Verification items for the finished model (mm, model axes). Face numbers are marked on the shaded views. A direction names the side the tool comes from. Round coordinates to 2 decimals unless told otherwise and drop trailing zeros. Loops run counter-clockwise (first coordinate to the right, second up) from the corner with the lowest first, then second, coordinate; pieces in that order, holes last. Notation, with made-up numbers: (-27.75, 30) - (24.25, 30) arc R17 ccw to (24.25, 62) - close; hole circle Ø1 at (59, 89.25). An arc over 180 degrees is marked (long way). Use a Markdown table: item, result. Add a question column.
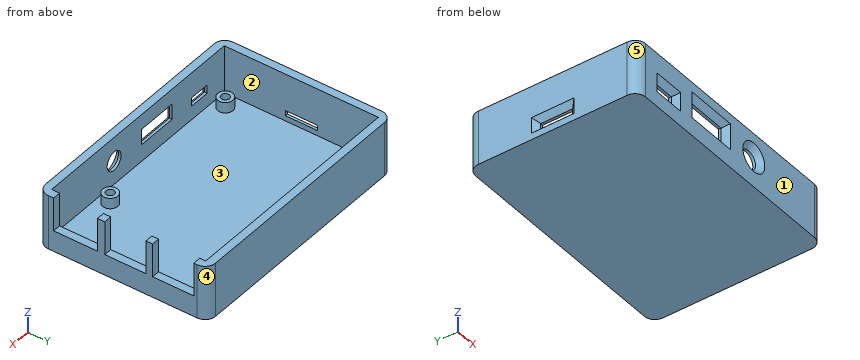
```python
from build123d import *

# Parameters (mm, degrees)
BASE_SKETCH_W               = 93
BASE_SKETCH_H               = 64
BASE_DEPTH                  = 2.5
WALLS_SKETCH_W              = 93
WALLS_SKETCH_H              = 64
WALLS_SKETCH_W_2            = 87
WALLS_SKETCH_H_2            = 58
WALLS_DEPTH                 = 18
FRONT_CONNECTORS_REACH      = 102.465
FRONT_CONNECTORS_SKETCH_W   = 12.6
FRONT_CONNECTORS_SKETCH_H   = 16.5
FRONT_CONNECTORS_SKETCH_H_2 = 15.5
SIDE_CONNECTORS_REACH       = 83.722
SIDE_CONNECTORS_SKETCH_R    = 3.5
SIDE_CONNECTORS_SKETCH_W    = 8
SIDE_CONNECTORS_SKETCH_H    = 3.2
SIDE_CONNECTORS_SKETCH_W_2  = 15.3
SIDE_CONNECTORS_SKETCH_H_2  = 5.9
SIDE_CONNECTORS_ANGLE_SIZE  = 2
SD_SLOT_REACH               = 102.465
SD_SLOT_SKETCH_W            = 2
SD_SLOT_SKETCH_H            = 12
SD_SLOT_ANGLE_SIZE          = 2
MOUNT_PILLAR_SKETCH_R       = 2.85
MOUNT_PILLARS_DEPTH         = 4
INSERT_NUT_HOLES_D          = 3.1
INSERT_NUT_HOLES_DEPTH      = 5
INSERT_NUT_HOLES_TIP        = 0.931333959
ZAOBLIT2_R                  = 4


with BuildPart() as part:
    # Base sketch → Base (new body)
    with BuildSketch(Plane.XY):
        Rectangle(BASE_SKETCH_W, BASE_SKETCH_H)
    extrude(amount=BASE_DEPTH)

    # Walls sketch → Walls (add)
    with BuildSketch(Plane.XY.offset(2.5)):
        Rectangle(WALLS_SKETCH_W, WALLS_SKETCH_H)
        Rectangle(WALLS_SKETCH_W_2, WALLS_SKETCH_H_2, mode=Mode.SUBTRACT)
    extrude(amount=WALLS_DEPTH)

    # Front connectors sketch → Front connectors (cut, up to next)
    with BuildSketch(Plane(origin=(46.5, 0, 0), x_dir=(0, 0, -1), z_dir=(1, 0, 0)), mode=Mode.PRIVATE) as front_connectors_sk1:
        with Locations((-14.2, -17.75)):
            Rectangle(FRONT_CONNECTORS_SKETCH_W, FRONT_CONNECTORS_SKETCH_H)
    front_connectors_tool1 = extrude(front_connectors_sk1.sketch, amount=-FRONT_CONNECTORS_REACH, mode=Mode.PRIVATE) & part.part
    # Front connectors sketch → Front connectors (cut, up to next)
    with BuildSketch(Plane(origin=(46.5, 0, 0), x_dir=(0, 0, -1), z_dir=(1, 0, 0)), mode=Mode.PRIVATE) as front_connectors_sk2:
        with Locations((-14.2, 1)):
            Rectangle(FRONT_CONNECTORS_SKETCH_W, FRONT_CONNECTORS_SKETCH_H_2)
    front_connectors_tool2 = extrude(front_connectors_sk2.sketch, amount=-FRONT_CONNECTORS_REACH, mode=Mode.PRIVATE) & part.part
    # Front connectors sketch → Front connectors (cut, up to next)
    with BuildSketch(Plane(origin=(46.5, 0, 0), x_dir=(0, 0, -1), z_dir=(1, 0, 0)), mode=Mode.PRIVATE) as front_connectors_sk3:
        with Locations((-14.2, 19)):
            Rectangle(FRONT_CONNECTORS_SKETCH_W, FRONT_CONNECTORS_SKETCH_H_2)
    front_connectors_tool3 = extrude(front_connectors_sk3.sketch, amount=-FRONT_CONNECTORS_REACH, mode=Mode.PRIVATE) & part.part
    add(front_connectors_tool1.solids().sort_by_distance((46.5, -17.75, 14.2))[0], mode=Mode.SUBTRACT)
    add(front_connectors_tool2.solids().sort_by_distance((46.5, 1, 14.2))[0], mode=Mode.SUBTRACT)
    add(front_connectors_tool3.solids().sort_by_distance((46.5, 19, 14.2))[0], mode=Mode.SUBTRACT)

    # Side connectors sketch → Side connectors (cut, up to next)
    with BuildSketch(Plane.XZ.offset(32), mode=Mode.PRIVATE) as side_connectors_sk1:
        with Locations(Location((12, 11.4, 0), (0, 0, 270))):
            Circle(SIDE_CONNECTORS_SKETCH_R)
    side_connectors_tool1 = extrude(side_connectors_sk1.sketch, amount=-SIDE_CONNECTORS_REACH, mode=Mode.PRIVATE) & part.part
    # Side connectors sketch → Side connectors (cut, up to next)
    with BuildSketch(Plane.XZ.offset(32), mode=Mode.PRIVATE) as side_connectors_sk2:
        with Locations((-30.9, 9.3)):
            Rectangle(SIDE_CONNECTORS_SKETCH_W, SIDE_CONNECTORS_SKETCH_H)
    side_connectors_tool2 = extrude(side_connectors_sk2.sketch, amount=-SIDE_CONNECTORS_REACH, mode=Mode.PRIVATE) & part.part
    # Side connectors sketch → Side connectors (cut, up to next)
    with BuildSketch(Plane.XZ.offset(32), mode=Mode.PRIVATE) as side_connectors_sk3:
        with Locations((-9.5, 11.85)):
            Rectangle(SIDE_CONNECTORS_SKETCH_W_2, SIDE_CONNECTORS_SKETCH_H_2)
    side_connectors_tool3 = extrude(side_connectors_sk3.sketch, amount=-SIDE_CONNECTORS_REACH, mode=Mode.PRIVATE) & part.part
    add(side_connectors_tool1.solids().sort_by_distance((12, -32, 11.4))[0], mode=Mode.SUBTRACT)
    add(side_connectors_tool2.solids().sort_by_distance((-30.9, -32, 9.3))[0], mode=Mode.SUBTRACT)
    add(side_connectors_tool3.solids().sort_by_distance((-9.5, -32, 11.85))[0], mode=Mode.SUBTRACT)

    # Side connectors angle
    side_connectors_angle_edges = [part.edges().sort_by_distance(p)[0] for p in [
        (-9.5, -32, 8.9),
        (-1.85, -32, 11.85),
        (-9.5, -32, 14.8),
        (-17.15, -32, 11.85),
        (12, -32, 14.9),
        (-34.9, -32, 9.3),
        (-30.9, -32, 7.7),
        (-26.9, -32, 9.3),
        (-30.9, -32, 10.9),
    ]]
    chamfer(side_connectors_angle_edges, length=SIDE_CONNECTORS_ANGLE_SIZE)

    # SD slot sketch → SD slot (cut, up to next)
    with BuildSketch(Plane.ZY.offset(46.5), mode=Mode.PRIVATE) as sd_slot_sk1:
        with Locations((5.5, 0)):
            Rectangle(SD_SLOT_SKETCH_W, SD_SLOT_SKETCH_H)
    sd_slot_tool1 = extrude(sd_slot_sk1.sketch, amount=-SD_SLOT_REACH, mode=Mode.PRIVATE) & part.part
    add(sd_slot_tool1.solids().sort_by_distance((-46.5, 0, 5.5))[0], mode=Mode.SUBTRACT)

    # SD slot angle
    sd_slot_angle_edges = [part.edges().sort_by_distance(p)[0] for p in [
        (-46.5, 0, 6.5),
        (-46.5, -6, 5.5),
        (-46.5, 6, 5.5),
        (-46.5, 0, 4.5),
    ]]
    chamfer(sd_slot_angle_edges, length=SD_SLOT_ANGLE_SIZE)

    # Mount pillar sketch → Mount pillars (add)
    with BuildSketch(Plane.XY.offset(2.5)):
        with Locations((-38, -24.5)):
            Circle(MOUNT_PILLAR_SKETCH_R)
        with Locations((20, -24.5)):
            Circle(MOUNT_PILLAR_SKETCH_R)
        with Locations((20, 24.5)):
            Circle(MOUNT_PILLAR_SKETCH_R)
        with Locations((-38, 24.5)):
            Circle(MOUNT_PILLAR_SKETCH_R)
    extrude(amount=MOUNT_PILLARS_DEPTH)

    # Insert nut holes
    with Locations(Plane.XY.offset(6.5)):
        with Locations((-38, 24.5), (20, 24.5), (20, -24.5), (-38, -24.5)):
            Hole(INSERT_NUT_HOLES_D / 2, depth=INSERT_NUT_HOLES_DEPTH)
            with Locations((0, 0, -(INSERT_NUT_HOLES_DEPTH + INSERT_NUT_HOLES_TIP / 2))):  # 118° drill point
                Cone(0, INSERT_NUT_HOLES_D / 2, INSERT_NUT_HOLES_TIP, mode=Mode.SUBTRACT)

    # Zaoblit2
    zaoblit2_edges = [part.edges().sort_by_distance(p)[0] for p in [
        (46.5, 32, 10.25),
        (46.5, -32, 10.25),
        (-46.5, -32, 10.25),
        (-46.5, 32, 10.25),
    ]]
    fillet(zaoblit2_edges, radius=ZAOBLIT2_R)


solid = part.part
```
Q1. Section check D-D on y = -12.5. Record the cut outline in (x, z).
Q2. Section check A-A on y = 1. Record the cut outline in (x, z), plus the area to 3 significant figures.
Q3. Section check C-C on z = 19.25. Record the cut outline in (x, y).
Q4. Section check B-B on x = 12. Record the cut outline in (y, z), plus the area to 3 significant figures.
Q5. Go/stop test with flat-tipped pins: pin 1 Ø0.8 at (y, z) = (-29.5, 12) entering from -X; pin 2 Ø6 at (y, z) = (4, 14.5) entering from +X; pin 3 Ø2.5 at (x, z) = (45, 12.5) entering from +Y. Record where each tip stops, or that it passes through.
Q6. Set-up check for the marked faces 1 and 2: record each of +Z, -Z, +X, -X, +Y, -Y from which the full face is reachable in a straight line by a thin tool's end or side.
Q7. Thickness scan on line 1 along Y through (x, z) = (-38, 3.7); line 2 along Y through (x, z) = (30, 17.75); line 3 along X through (y, z) = (11.5, 5.5). Record the ranges inside material, lowest first.
Q8. Release check for a two-part mould opening along X. For the marked faces 3, 4 and 5 record: +X half, -X half, draft (parallel to the pull), parting line (faces both ways), or undercut.
Determined:
| question | item | result |
|---|---|---|
| 1 | outline | (-46.5, 0) - (46.5, 0) - (46.5, 7.9) - (43.5, 7.9) - (43.5, 2.5) - (-43.5, 2.5) - (-43.5, 20.5) - (-46.5, 20.5) - close |
| 2 | outline | (-46.5, 0) - (46.5, 0) - (46.5, 7.9) - (43.5, 7.9) - (43.5, 2.5) - (-43.5, 2.5) - (-43.5, 4.5) - (-44.5, 4.5) - (-46.5, 2.5) - close; (-46.5, 8.5) - (-44.5, 6.5) - (-43.5, 6.5) - (-43.5, 20.5) - (-46.5, 20.5) - close |
| 2 | area | 293 mm² |
| 3 | outline | (-46.5, -28) arc R4 ccw to (-42.5, -32) - (42.5, -32) arc R4 ccw to (46.5, -28) - (46.5, -26) - (43.5, -26) - (43.5, -29) - (-43.5, -29) - (-43.5, 29) - (43.5, 29) - (43.5, 26.75) - (46.5, 26.75) - (46.5, 28) arc R4 ccw to (42.5, 32) - (-42.5, 32) arc R4 ccw to (-46.5, 28) - close; (43.5, -9.5) - (46.5, -9.5) - (46.5, -6.75) - (43.5, -6.75) - close; (43.5, 8.75) - (46.5, 8.75) - (46.5, 11.25) - (43.5, 11.25) - close |
| 4 | outline | (-32, 0) - (32, 0) - (32, 20.5) - (29, 20.5) - (29, 2.5) - (-29, 2.5) - (-29, 7.9) - (-30, 7.9) - (-32, 5.9) - close; (-32, 16.9) - (-30, 14.9) - (-29, 14.9) - (-29, 20.5) - (-32, 20.5) - close |
| 4 | area | 243 mm² |
| 5 | pin 1 | stops at x = -46.35 |
| 5 | pin 2 | stops at x = -43.5 |
| 5 | pin 3 | stops at y = 31.8 |
| 6 | face 1 | +Z, -Z, +X, -X, -Y |
| 6 | face 2 | +Z |
| 7 | line 1 | y = -32 to -29, -27.35 to -26.05, -22.95 to -21.65, 21.65 to 22.95, 26.05 to 27.35, 29 to 32 |
| 7 | line 2 | y = -32 to -29, 29 to 32 |
| 7 | line 3 | x = -46.5 to -43.5, 43.5 to 46.5 |
| 8 | face 3 | undercut |
| 8 | face 4 | +X half |
| 8 | face 5 | -X half |
